Can you work these out from the model? Positions are in its coordinate system, mm. Face numbers are marked on the shaded views. A direction names the side the tool comes from. Give positions to 0.01 mm unless a question says otherwise; leave off trailing zeros. Order: outer loops, then holes, each group sorted by start corner. A loop starts at its lowest first (then second) coordinate and runs counter-clockwise, first axis right, second up. Notation, with made-up numbers: M 71,22 L 114,22 A29 ccw 114,58 Z; hole C -39,-28 d8. An arc over 180 degrees is marked long. Use a Markdown table: item, result. Add a question column.
from build123d import *

# Parameters (mm, degrees)
SKETCH1_W           = 762
SKETCH1_H           = 1828.8
BOSS_EXTRUDE1_DEPTH = 152.4
SKETCH2_W           = 711.2
SKETCH2_H           = 1778
CUT_EXTRUDE3_DEPTH  = 127
SKETCH10_W          = 101.6
SKETCH10_H          = 101.6
CUT_EXTRUDE4_DEPTH  = 12.7


with BuildPart() as part:
    # Sketch1 → Boss-Extrude1 (new body)
    with BuildSketch(Plane.XY):
        with Locations((-1498.701019621, -163.505851304)):
            Rectangle(SKETCH1_W, SKETCH1_H)
    extrude(amount=BOSS_EXTRUDE1_DEPTH)

    # Sketch2 → Cut-Extrude3 (cut)
    with BuildSketch(Plane.XY.offset(152.4)):
        with Locations((-1498.701019621, -163.505851304)):
            Rectangle(SKETCH2_W, SKETCH2_H)
    extrude(amount=-CUT_EXTRUDE3_DEPTH, mode=Mode.SUBTRACT)

    # Sketch10 → Cut-Extrude4 (cut)
    with BuildSketch(Plane.XY.offset(25.4)):
        with Locations((-1498.701019621, 306.394148696)):
            Rectangle(SKETCH10_W, SKETCH10_H)
        with Locations((-1498.701019621, -163.505851304)):
            Rectangle(SKETCH10_W, SKETCH10_H)
        with Locations((-1498.701019621, -633.405851304)):
            Rectangle(SKETCH10_W, SKETCH10_H)
    extrude(amount=-CUT_EXTRUDE4_DEPTH, mode=Mode.SUBTRACT)


solid = part.part
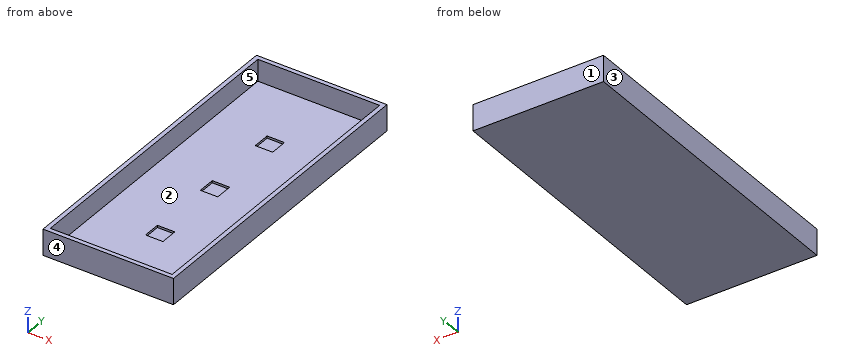
1. On a 3-axis mill with a long thin cutter (end or side, diameter ignored), from which of +Z, -Z, +X, -X, +Y, -Y can I reach the whole of each face in a straight line? I mean the marked faces 1 and 2. Say none if no direction works.
2. If we section it at A-A, the plane z = 119.5: List the corners of the cut face in (x, y) for me, then the cut area to 3 significant figures.
3. Will these pins go through, and if not, where does the flat tip stop? pin 1 (4 mm diameter, centred on x = -1470, y = -303, fed in from +Z); pin 2 (1 mm diameter, centred on x = -1779.5, y = 544.5, fed in from -Z).
4. If we section it at C-C, the plane x = -1391: List the corners of the cut face in (y, z) for me.
5. If we section it at D-D, the plane y = -134: List the corners of the cut face in (x, z) for me, then the cut area to 3 significant figures.
6. I need wall thicknesses on L1, parallel to Y at x = -1274, z = 68.5; L2, parallel to X at y = -324, z = 125.5; L3, parallel to X at y = -198, z = 20.5. Which ranges of each line are inside material? Lowest first, please. Write a range as [from, to].
7. We'd pull the mould along Y, two halves only. Please class the marked faces 3, 4 and 5: +Y half, -Y half, draft (parallel to the pull), parting line (faces both ways), or undercut.
8. If we section it at B-B, the plane y = -729: List the corners of the cut face in (x, z) for me, then the cut area to 3 significant figures.
Geometry results:
| question | item | result |
|---|---|---|
| 1 | face 1 | +Z, -Z, +X, -X, +Y |
| 1 | face 2 | +Z |
| 2 | outline | M -1879.7,-1077.91 L -1117.7,-1077.91 L -1117.7,750.89 L -1879.7,750.89 Z; hole M -1854.3,-1052.51 L -1143.1,-1052.51 L -1143.1,725.49 L -1854.3,725.49 Z |
| 2 | area | 129,000 mm^2 |
| 3 | pin 1 | stops at z = 25.4 |
| 3 | pin 2 | stops at z = 0 |
| 4 | outline | M -1077.91,0 L 750.89,0 L 750.89,152.4 L 725.49,152.4 L 725.49,25.4 L -1052.51,25.4 L -1052.51,152.4 L -1077.91,152.4 Z |
| 5 | outline | M -1879.7,0 L -1117.7,0 L -1117.7,152.4 L -1143.1,152.4 L -1143.1,25.4 L -1447.9,25.4 L -1447.9,12.7 L -1549.5,12.7 L -1549.5,25.4 L -1854.3,25.4 L -1854.3,152.4 L -1879.7,152.4 Z |
| 5 | area | 24,500 mm^2 |
| 6 | L1 | y = [-1077.91, -1052.51], [725.49, 750.89] |
| 6 | L2 | x = [-1879.7, -1854.3], [-1143.1, -1117.7] |
| 6 | L3 | x = [-1879.7, -1549.5], [-1447.9, -1117.7] |
| 7 | face 3 | draft |
| 7 | face 4 | -Y half |
| 7 | face 5 | undercut |
| 8 | outline | M -1879.7,0 L -1117.7,0 L -1117.7,152.4 L -1143.1,152.4 L -1143.1,25.4 L -1854.3,25.4 L -1854.3,152.4 L -1879.7,152.4 Z |
| 8 | area | 25,800 mm^2 |
